from build123d import *

# Parameters (mm, degrees)
F0_R     = 39.78873575
F0_R_2   = 34.78873575
F1_DEPTH = 26.1
F0_R_3   = 7
F0_R_4   = 3.5
F2_DEPTH = 4.9
F0_R_5   = 2.5
F3_DEPTH = 2
F4_DEPTH = 21
F6_START = 25
F5_W     = 19.6
F5_H     = 13
F6_DEPTH = 20
F7_START = 36.5
F5_W_2   = 21.5
F5_H_2   = 15.5
F7_DEPTH = 8.5
F8_START = 25
F8_DEPTH = 11.5
F9_START = 25
F9_DEPTH = 11.5


# Not quite as in the source:
# - a feature names something its author has since deleted; it is built from what else it names


with BuildPart() as f1:
    # F0 (on Top) → F1 (new body)
    with BuildSketch(Plane.XY):
        Circle(F0_R)
        Circle(F0_R_2, mode=Mode.SUBTRACT)
    extrude(amount=F1_DEPTH)

    # F0 (on Top) → F2 (join)
    with BuildSketch(Plane.XY):
        Circle(F0_R_2)
        with Locations((-20, 0)):
            Circle(F0_R_3, mode=Mode.SUBTRACT)
        Circle(F0_R_4, mode=Mode.SUBTRACT)
        Polygon((20, 4.1030999273), (20, 8), (25, 8), (25, 5), (25, -5), (25, -8), (20, -8), (20, -4.1030999273), align=None, mode=Mode.SUBTRACT)
    extrude(amount=F2_DEPTH)

    # F0 (on Top) → F3 (join)
    with BuildSketch(Plane.XY):
        Circle(F0_R_4)
        Circle(F0_R_5, mode=Mode.SUBTRACT)
    extrude(amount=F3_DEPTH)



with BuildPart() as f2:
    # F0 (on Top) → F2, piece 2 (new body)
    with BuildSketch(Plane.XY):
        Polygon((-24.1344178899, 2.3386082852), (-24.0925031294, -2.4112067799), (-19.9580852395, -4.7498150651), (-15.8655821101, -2.3386082852), (-15.9074968706, 2.4112067799), (-20.0419147605, 4.7498150651), align=None)
    extrude(amount=F2_DEPTH)


with BuildPart() as f1_1:
    add(f1.part)

    add(f2.part)  # F4 merges F2
    # F0 (on Top) → F4 (join)
    with BuildSketch(Plane.XY):
        with Locations((-20, 0)):
            Circle(F0_R_3)
        Polygon((-19.9580852395, -4.7498150651), (-24.0925031294, -2.4112067799), (-24.1344178899, 2.3386082852), (-20.0419147605, 4.7498150651), (-15.9074968706, 2.4112067799), (-15.8655821101, -2.3386082852), align=None, mode=Mode.SUBTRACT)
    extrude(amount=F4_DEPTH)

    # F5 (on Front) → F6 (cut)
    with BuildSketch(Plane.XZ.offset(F6_START)):
        with Locations((0, 11.4)):
            Rectangle(F5_W, F5_H)
    extrude(amount=F6_DEPTH, mode=Mode.SUBTRACT)

    # F5 (on Front) → F7 (cut)
    with BuildSketch(Plane.XZ.offset(F7_START)):
        with Locations((0, 11.4)):
            Rectangle(F5_W_2, F5_H_2)
        with Locations((0, 11.4)):
            Rectangle(F5_W, F5_H, mode=Mode.SUBTRACT)
    extrude(amount=F7_DEPTH, mode=Mode.SUBTRACT)

    # F5 (on Front) → F8 (join)
    with BuildSketch(Plane.XZ.offset(F8_START)):
        with Locations((0, 11.4)):
            Rectangle(F5_W_2, F5_H_2)
        with Locations((0, 11.4)):
            Rectangle(F5_W, F5_H, mode=Mode.SUBTRACT)
    extrude(amount=F8_DEPTH)

    # F5 (on Front) → F9 (join)
    with BuildSketch(Plane.XZ.offset(F9_START)):
        Polygon((-10.75, 3.65), (-10.75, 19.15), (10.75, 19.15), (10.75, 3.65), (12.25, 3.65), (12.25, 21), (-12.25, 21), (-12.25, 3.65), align=None)
    extrude(amount=F9_DEPTH)


solid = f1_1.part
Check sheet for the modelled part. Datum: model origin and axes. Units: mm. A direction names the side the tool comes from. Give positions to 0.01 mm unless a question says otherwise; leave off trailing zeros. Loops run counter-clockwise (first coordinate to the right, second up) from the corner with the lowest first, then second, coordinate; pieces in that order, holes last. Notation, with made-up numbers: M 0.5,-28 L 31.5,-28 A12 ccw 31.5,-24 Z; hole C 74.25,35.25 d10. An arc over 180 degrees is marked long. Use a Markdown table: item, result. Add a question column.
Q1. Scan lines: line 1 along Y through (x, z) = (0, 1.4); line 2 along Y through (x, z) = (0, 3.1); line 3 along X through (y, z) = (-30, 5.25). Record each from-to range of solid material in increasing order. Write a range as [from, to].
Q2. Sectioned sample at B-B, the plane x = 0. Record the cut outline in (y, z), then the cut area to 3 significant figures.
Q3. Tool access check on faces 1 (the flat face through (0, -31, 17.9)), 2 (the flat face through (-18.004, 3.597, 12.837)), 3 (the flat face through (22, 8, 2)). Record the directions out of +Z, -Z, +X, -X, +Y, -Y that give a thin tool (end or side, any length) a straight path to the whole face; none if there is none.
Q4. Sectioned sample at C-C, the plane y = 0. Record the cut outline in (x, z).
Q5. Go/stop test with flat-tipped pins: pin 1 (8 mm diameter, centred on x = -4.5, z = 10.5, fed in from +Y); pin 2 (1.5 mm diameter, centred on y = 21, z = 17.5, fed in from -X); pin 3 (10 mm diameter, centred on y = 8.5, z = 3.5, fed in from +X). Record where each tip stops, or that it passes through.
Q6. Sectioned sample at D-D, the plane x = 8.5. Record the cut outline in (y, z).
Q7. Sectioned sample at A-A, the plane z = 15.25. Record the cut outline in (x, y), then the cut area to 3 significant figures.
Q8. Mould release check, pull along X, two halves, no side actions. Record for faces 4 (the flat face through (-22.117, 3.527, 12.837)), 5 (the flat face through (0, -35, 26.1)), 6 (the cylindrical face through (-5.18, 39.45, 12.87)): pulls with the +X half, pulls with the -X half, needs draft (parallel to the pull), parting line crosses it, or undercut.
Verdict:
| question | item | result |
|---|---|---|
| 1 | line 1 | [-39.79, -2.5], [2.5, 39.79] |
| 1 | line 2 | [-39.79, -3.5], [3.5, 39.79] |
| 1 | line 3 | [-26.14, -17.61], [-12.25, -9.8], [9.8, 12.25], [17.61, 26.14] |
| 2 | outline | M -39.79,0 L -2.5,0 L -2.5,2 L -3.5,2 L -3.5,4.9 L -36.5,4.9 L -36.5,3.65 L -39.79,3.65 Z; M -39.79,19.15 L -36.5,19.15 L -36.5,17.9 L -25,17.9 L -25,21 L -34.79,21 L -34.79,26.1 L -39.79,26.1 Z; M 2.5,0 L 39.79,0 L 39.79,26.1 L 34.79,26.1 L 34.79,4.9 L 3.5,4.9 L 3.5,2 L 2.5,2 Z |
| 2 | area | 529 mm^2 |
| 3 | face 1 | -Y |
| 3 | face 2 | +Z |
| 3 | face 3 | +Z, -Z |
| 4 | outline | M -39.79,0 L -2.5,0 L -2.5,2 L -3.5,2 L -3.5,4.9 L -13,4.9 L -13,21 L -15.89,21 L -15.89,4.9 L -24.11,4.9 L -24.11,21 L -27,21 L -27,4.9 L -34.79,4.9 L -34.79,26.1 L -39.79,26.1 Z; M 2.5,0 L 20,0 L 20,4.9 L 3.5,4.9 L 3.5,2 L 2.5,2 Z; M 25,0 L 39.79,0 L 39.79,26.1 L 34.79,26.1 L 34.79,4.9 L 25,4.9 Z |
| 5 | pin 1 | y = 39.79 |
| 5 | pin 2 | x = -34.25 |
| 5 | pin 3 | x = 39.63 |
| 6 | outline | M -38.87,0 L 38.87,0 L 38.87,26.1 L 33.73,26.1 L 33.73,4.9 L -36.5,4.9 L -36.5,3.65 L -38.87,3.65 Z; M -38.87,19.15 L -36.5,19.15 L -36.5,17.9 L -25,17.9 L -25,21 L -33.73,21 L -33.73,26.1 L -38.87,26.1 Z |
| 7 | outline | C -20,0 d14; M -12.25,-32.56 A34.79 cw long 12.25,-32.56 L 12.25,-25 L 9.8,-25 L 9.8,-36.5 L 10.75,-36.5 L 10.75,-38.31 A39.79 ccw long -10.75,-38.31 L -10.75,-36.5 L -9.8,-36.5 L -9.8,-25 L -12.25,-25 Z; hole M -24.13,2.34 L -24.09,-2.41 L -19.96,-4.75 L -15.87,-2.34 L -15.91,2.41 L -20.04,4.75 Z |
| 7 | area | 1,200 mm^2 |
| 8 | face 4 | undercut |
| 8 | face 5 | needs draft |
| 8 | face 6 | parting line crosses it |
